Build history of the part. All positions in model axes, mm. Face numbers are marked on the shaded views. A direction names the side the tool comes from. Round coordinates to 2 decimals unless told otherwise and drop trailing zeros. Loops run counter-clockwise (first coordinate to the right, second up) from the corner with the lowest first, then second, coordinate; pieces in that order, holes last. Notation, with made-up numbers: (49, 43.25) - (62, 43.25) arc R23 ccw to (62, 70.25) - close; hole circle Ø1 at (2, 57). An arc over 180 degrees is marked (long way). Answer as CSV lines item,"result". Start each with the question number.
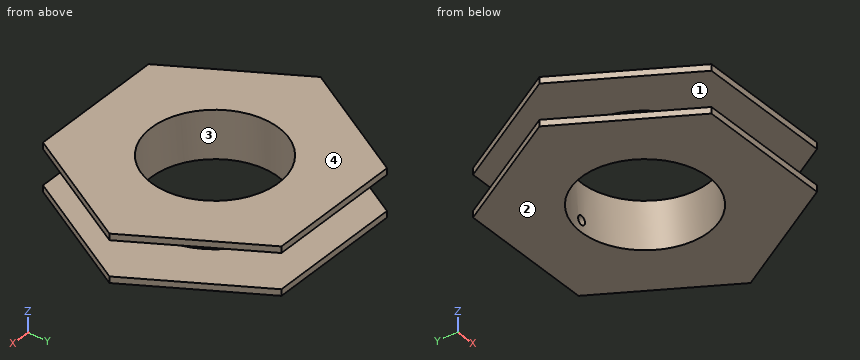
```python
from build123d import *

# Parameters (mm, degrees)
F1_DEPTH = 7.62
F2_R     = 10.16
F3_DEPTH = 25.4
F5_R     = 11.43
F6_DEPTH = 5.588
F7_R     = 0.718054
F8_DEPTH = 25.4


with BuildPart() as f1:
    # F0 (on Top) → F1 (new body)
    with BuildSketch(Plane.XY):
        Polygon((10.998523, 19.05), (-10.998523, 19.05), (-21.997045, 0), (-10.998523, -19.05), (10.998523, -19.05), (21.997045, 0), align=None)
    extrude(amount=F1_DEPTH)

    # F2 (on face) → F3 (cut)
    with BuildSketch(Plane(origin=(0, 0, 0), x_dir=(1, 0, 0), z_dir=(0, 0, -1))):
        Circle(F2_R)
    extrude(amount=-F3_DEPTH, mode=Mode.SUBTRACT)

    # F5 (on offset) → F6 (cut)
    with BuildSketch(Plane.XY.offset(1.016)):
        Polygon((10.998523, -19.05), (21.997045, 0), (10.998523, 19.05), (-10.998523, 19.05), (-21.997045, 0), (-10.998523, -19.05), align=None)
        Circle(F5_R, mode=Mode.SUBTRACT)
    extrude(amount=F6_DEPTH, mode=Mode.SUBTRACT)

    # F7 (on Front) → F8 (cut)
    with BuildSketch(Plane.XZ):
        with Locations((0, 1.871332)):
            Circle(F7_R)
    extrude(amount=-F8_DEPTH, mode=Mode.SUBTRACT)


solid = f1.part
```
Q1. Wall check: probe 1 along Z at (x, y) = (10.5, -7); probe 2 along Y at (x, z) = (0, 5); probe 3 along Z at (x, y) = (0, 11.15). Give the ranges that are in metal, low to high. Write a range as [from, to].
Q2. Pin check, flat tips, straight feed: pin 1 Ø4 at (y, z) = (6, 2) entering from +X; pin 2 Ø1.5 at (y, z) = (-6.5, 1) entering from -X; pin 3 Ø1.1 at (x, z) = (0, 1.87) entering from +Y. Stop position of each tip, or through.
Q3. Tool access for the marked faces 1 and 2: list every direction of +Z, -Z, +X, -X, +Y, -Y with a clear straight run to the whole face (end or side of a thin tool).
Q4. Band-saw the part on B-B, the plane y = -7. List the corners of the cut face in (x, z), then the cut area to 3 significant figures.
Q5. Band-saw the part on A-A, the plane x = 0. List the corners of the cut face in (y, z).
Q6. Band-saw the part on D-D, the plane y = -15.5. List the corners of the cut face in (x, z).
Q7. Band-saw the part on C-C, the plane x = -15.5. List the corners of the cut face in (y, z), then the cut area to 3 significant figures.
Q8. Two-plate mould, pull along Y, no slides. Class the marked faces 3 and 4: released by +Y, released by -Y, zero draft, split by the parting line, or undercut.
Reported:
1,probe 1,"z = [0, 1.02], [6.6, 7.62]"
1,probe 2,"y = [-11.43, -10.16], [10.16, 11.43]"
1,probe 3,"z = [0, 1.15], [2.59, 7.62]"
2,pin 1,"stops at x = 19.54"
2,pin 2,"stops at x = -18.68"
2,pin 3,"stops at y = -10.15"
3,face 1,"none"
3,face 2,"-Z, +X, -X, +Y, -Y"
4,outline,"(-17.96, 0) - (-7.36, 0) - (-7.36, 7.62) - (-17.96, 7.62) - (-17.96, 6.6) - (-9.04, 6.6) - (-9.04, 1.02) - (-17.96, 1.02) - close; (7.36, 0) - (17.96, 0) - (17.96, 1.02) - (9.04, 1.02) - (9.04, 6.6) - (17.96, 6.6) - (17.96, 7.62) - (7.36, 7.62) - close"
4,area,"61.7 mm2"
5,outline,"(-19.05, 0) - (-10.16, 0) - (-10.16, 7.62) - (-19.05, 7.62) - (-19.05, 6.6) - (-11.43, 6.6) - (-11.43, 1.02) - (-19.05, 1.02) - close; (10.16, 0) - (19.05, 0) - (19.05, 1.02) - (11.43, 1.02) - (11.43, 1.15) - (10.16, 1.15) - close; (10.16, 2.59) - (11.43, 2.59) - (11.43, 6.6) - (19.05, 6.6) - (19.05, 7.62) - (10.16, 7.62) - close"
6,outline,"(-13.05, 0) - (13.05, 0) - (13.05, 1.02) - (-13.05, 1.02) - close; (-13.05, 6.6) - (13.05, 6.6) - (13.05, 7.62) - (-13.05, 7.62) - close"
7,outline,"(-11.25, 0) - (11.25, 0) - (11.25, 1.02) - (-11.25, 1.02) - close; (-11.25, 6.6) - (11.25, 6.6) - (11.25, 7.62) - (-11.25, 7.62) - close"
7,area,"45.7 mm2"
8,face 3,"undercut"
8,face 4,"zero draft"
